Work out the finished part from the listing and answer in its coordinate system (mm). A direction names the side the tool comes from. Give positions to 0.01 mm unless a question says otherwise; leave off trailing zeros. Loops run counter-clockwise (first coordinate to the right, second up) from the corner with the lowest first, then second, coordinate; pieces in that order, holes last. Notation, with made-up numbers: (76.25, -38) - (85.25, -38) arc R14 cw to (85.25, -33) - close; hole circle Ø11 at (59, -22.75). An arc over 180 degrees is marked (long way). One line per question, with ' | ' between items. Start each with the question number.
1. Section A-A (y = 472.5) is taken. Determine the outline of the cut face in (x, z).
2. Section B-B (x = 74) is taken. Determine the outline of the cut face in (y, z), plus the area to 3 significant figures.
3. Each of these flat-tipped pins is pushed along its axis until it touches: pin 1 (20 mm diameter, centred on x = 150.5, y = 454.5, fed in from +Z); pin 2 (12 mm diameter, centred on x = 135, y = 374, fed in from +Z). Where does it stop, or does it pass through?
4. Section C-C (y = 455) is taken. Determine the outline of the cut face in (x, z), plus the area to 3 significant figures.
5. Which of the six approach directions +Z, -Z, +X, -X, +Y, -Y give full straight-line access (tool end or side, diameter ignored) to faces 1 (the face through (151.51, 464.52, 161.19)), 2 (the face through (-4.05, 446.31, 175.85)), 3 (the face through (147, 454, 165.5)), 4 (the face through (0.5, 437.4, 171.5))?
6. Find the intervals of material crossed by line 1 (Z direction, x = 34, y = 467.5), in increasing order.
from build123d import *

# Parameters (mm, degrees)
SKETCH016_W  = 195
SKETCH016_H  = 127
PAD012_DEPTH = 157
PAD013_DEPTH = 8.5
PAD014_DEPTH = 21


with BuildPart() as part:
    # Sketch016 → Pad012 (new body)
    with BuildSketch(Plane.XY):
        with Locations((97.5, -63.5)):
            Rectangle(SKETCH016_W, SKETCH016_H)
    extrude(amount=PAD012_DEPTH)

    # Sketch017 (on Face6 of Pad012) → Pad013 (join)
    with BuildSketch(Plane.XY.offset(157)):
        with BuildLine():
            ThreePointArc((29.6383749954, -24.6988937525), (14.6988937525, -20.3616250046), (10.3616250046, -35.3011062475))
            Line((10.3616250046, -35.3011062475), (20, -52.825424421))
            Line((20, -52.825424421), (39.2767499909, -42.223211926))
            Line((39.2767499909, -42.223211926), (29.6383749954, -24.6988937525))
        make_face()
        with BuildLine():
            Line((175, -52.825424421), (184.6383749954, -35.3011062475))
            ThreePointArc((184.6383749954, -35.3011062475), (180.3011062475, -20.3616250046), (165.3616250046, -24.6988937525))
            Line((165.3616250046, -24.6988937525), (155.7232500091, -42.223211926))
            Line((155.7232500091, -42.223211926), (175, -52.825424421))
        make_face()
    extrude(amount=PAD013_DEPTH)

    # Sketch018 (on Face15 of Pad013) → Pad014 (join)
    with BuildSketch(Plane.XY.offset(165.5)):
        Polygon((20, -52.825424421), (39.2767499909, -42.223211926), (34.4575624932, -33.4610528393), (15.1808125023, -44.0632653343), align=None)
        Polygon((155.7232500091, -42.223211926), (175, -52.825424421), (179.8191874977, -44.0632653343), (160.5424375068, -33.4610528393), align=None)
    extrude(amount=PAD014_DEPTH)


with BuildPart() as part_1:
    # Body005 placement: moved
    add(part.part.moved(Location((-29, 485, 0))))


solid = part_1.part
Conclusion:
1) outline: (-29, 0) - (166, 0) - (166, 157) - (-29, 157) - close
2) outline: (358, 0) - (485, 0) - (485, 157) - (358, 157) - close | area: 19,900 mm²
3) pin 1: z = 165.5 | pin 2: z = 157
4) outline: (-29, 0) - (166, 0) - (166, 157) - (157, 157) - (157, 165.5) - (133.45, 165.5) - (133.45, 157) - (3.55, 157) - (3.55, 165.5) - (-20, 165.5) - (-20, 157) - (-29, 157) - close | area: 31,000 mm²
5) face 1: +Z | face 2: +Z, -X, +Y | face 3: +Z, +X, +Y | face 4: +Z, -Y
6) line 1: 0 to 157
